Work out the finished part from the listing and answer in its coordinate system (mm). A direction names the side the tool comes from. Round coordinates to 2 decimals unless told otherwise and drop trailing zeros. Order: outer loops, then holes, each group sorted by start corner. A loop starts at its lowest first (then second) coordinate and runs counter-clockwise, first axis right, second up. Notation, with made-up numbers: (47, -17.5) -> (93, -17.5) arc R18 cw to (93, -2.5) -> close; hole circle Ø1 at (10, 81.25). An arc over 180 degrees is marked (long way). Use a Markdown table: item, result. Add a question column.
Item 1: Find the intervals of material crossed by L1, parallel to X at y = 0, z = 7.5; L2, parallel to Y at x = 0, z = 4.25; L3, parallel to X at y = 25, z = 1.75, in increasing order. Write a range as [from, to].
Item 2: A cutting plane is placed at D-D, the plane x = -15. Determine the outline of the cut face in (y, z).
Item 3: A cutting plane is placed at A-A, the plane y = 0. Determine the outline of the cut face in (x, z).
Item 4: A cutting plane is placed at C-C, the plane y = 33.5. Determine the outline of the cut face in (x, z).
Item 5: For a pull along X with two mould halves and no side action, classify faces 3 (the flat face through (3.933, 35, 5)), 4 (the flat face through (-3.933, 34, 5)), 5 (the cylindrical face through (0.1, 45.25, 5.07)) as +X half, -X half, draft (parallel to the pull), parting line (faces both ways), or undercut.
Item 6: Flat-ended cylindrical pins translate along their axes: P1, Ø2, axis at y = 41.5, z = 5, coming from the +X side; P2, Ø16, axis at x = 0, y = 0, coming from the -Z side; P3, Ø3, axis at x = 10, z = 7, coming from the -Y side; P4, Ø1.5, axis at x = 1.5, z = 3.5, coming from the -Y side. Find the tip coordinate at first contact, or state that the pin passes through.
Item 7: A cutting plane is placed at B-B, the plane z = 5.5. Determine the outline of the cut face in (x, y).
Item 8: A tool of negligible diameter and unlimited length cuts with its end or side. For faces 1 (the cylindrical face through (3.505, 50.601, 5.07)), 2 (the flat face through (0.251, 50, 5)), from which of +Z, -Z, +X, -X, +Y, -Y can it reach the whole face along a straight path? Write none if from no direction.
from build123d import *

# Parameters (mm, degrees)
BOSS_EXTRUDE1_DEPTH = 10
FILLET1_R           = 1.5
FILLET2_R           = 3
CUT_EXTRUDE1_DEPTH  = 10


with BuildPart() as part:
    # Sketch1 → Boss-Extrude1 (new body)
    with BuildSketch(Plane.XY):
        with BuildLine():
            Line((3.932919229, 51.05226265), (3.932919229, 16.949694579))
            ThreePointArc((3.932919229, 16.949694579), (15.446427165, 8.010486117), (16.11997205, -6.550305421))
            Line((16.11997205, -6.550305421), (11.747169825, -6.550305421))
            ThreePointArc((11.747169825, -6.550305421), (0, 13.45), (-11.747169825, -6.550305421))
            Line((-11.747169825, -6.550305421), (-16.11997205, -6.550305421))
            ThreePointArc((-16.11997205, -6.550305421), (-15.446427165, 8.010486117), (-3.932919229, 16.949694579))
            Line((-3.932919229, 16.949694579), (-3.932919229, 51.05226265))
            Line((-3.932919229, 51.05226265), (3.932919229, 51.05226265))
        make_face()
    extrude(amount=BOSS_EXTRUDE1_DEPTH)

    # Fillet1
    fillet1_edges = [part.edges().sort_by_distance(p)[0] for p in [
        (-3.932919229, 51.05226265, 5),
        (3.932919229, 51.05226265, 5),
    ]]
    fillet(fillet1_edges, radius=FILLET1_R)

    # Fillet2
    fillet2_edges = [part.edges().sort_by_distance(p)[0] for p in [
        (-3.932919229, 16.949694579, 5),
        (3.932919229, 16.949694579, 5),
    ]]
    fillet(fillet2_edges, radius=FILLET2_R)

    # Sketch3 → Cut-Extrude1 (cut)
    with BuildSketch(Plane.XY.offset(10)):
        with BuildLine():
            Line((-0.269258516, 49.33121061), (-0.269258516, 51.05226265))
            Line((-0.269258516, 51.05226265), (0.251212815, 51.05226265))
            Line((0.251212815, 51.05226265), (0.251212815, 49.333520115))
            ThreePointArc((0.251212815, 49.333520115), (0.009096443, 45.248990685), (-0.269258516, 49.33121061))
        make_face()
    extrude(amount=-CUT_EXTRUDE1_DEPTH, mode=Mode.SUBTRACT)


solid = part.part
Reported:
| question | item | result |
|---|---|---|
| 1 | L1 | [-17.4, -13.45], [13.45, 17.4] |
| 1 | L2 | [13.45, 45.25] |
| 1 | L3 | [-3.93, 3.93] |
| 2 | outline | (-6.55, 0) -> (8.82, 0) -> (8.82, 10) -> (-6.55, 10) -> close |
| 3 | outline | (-17.4, 0) -> (-13.45, 0) -> (-13.45, 10) -> (-17.4, 10) -> close; (13.45, 0) -> (17.4, 0) -> (17.4, 10) -> (13.45, 10) -> close |
| 4 | outline | (-3.93, 0) -> (3.93, 0) -> (3.93, 10) -> (-3.93, 10) -> close |
| 5 | face 3 | +X half |
| 5 | face 4 | -X half |
| 5 | face 5 | undercut |
| 6 | P1 | x = 3.93 |
| 6 | P2 | through |
| 6 | P3 | y = 6.98 |
| 6 | P4 | y = 13.26 |
| 7 | outline | (-16.12, -6.55) -> (-11.75, -6.55) arc R13.45 cw (long way) to (11.75, -6.55) -> (16.12, -6.55) arc R17.4 ccw to (5.91, 16.36) arc R3 cw to (3.93, 19.19) -> (3.93, 49.55) arc R1.5 ccw to (2.43, 51.05) -> (0.25, 51.05) -> (0.25, 49.33) arc R2.05 cw (long way) to (-0.27, 49.33) -> (-0.27, 51.05) -> (-2.43, 51.05) arc R1.5 ccw to (-3.93, 49.55) -> (-3.93, 19.19) arc R3 cw to (-5.91, 16.36) arc R17.4 ccw to start |
| 8 | face 1 | +Z, -Z, +X, +Y |
| 8 | face 2 | +Z, -Z, +Y |
